Source: CAD feature listing. Evaluate the final solid. Frame: model axes, mm. A direction names the side the tool comes from. Give positions to 0.01 mm unless a question says otherwise; leave off trailing zeros. Order: outer loops, then holes, each group sorted by start corner. A loop starts at its lowest first (then second) coordinate and runs counter-clockwise, first axis right, second up. Notation, with made-up numbers: M 80.25,62 L 119.25,62 A23 ccw 119.25,72 Z; hole C 70.25,73.5 d4. An arc over 180 degrees is marked long. Answer as a JSON object with one key per item and string values. Group by question number.
1. Set-up query: faces 5 (the flat face through (37.5, 40, -10)), 6 (the flat face through (41, 122, -3)), 7 (the flat face through (45, 117, 1)). Return all of +Z, -Z, +X, -X, +Y, -Y with unobstructed straight access to the full face (end or side cutting, diameter ignored); none if empty.
2. Section query C-C (z = -20.5). Output: boundary loops of the cut face in (x, y).
3. Section query B-B (x = 54). Output: boundary loops of the cut face in (y, z), plus the area to 3 significant figures.
4. Material intervals for L1, parallel to Y at x = 50.5, z = 1.75; L2, parallel to Z at x = 24, y = 7; L3, parallel to X at y = 113, z = 4, sorted ascending. Write a range as [from, to].
5. Section query D-D (y = 24). Output: boundary loops of the cut face in (x, z), plus the area to 3 significant figures.
6. Pull-direction query (Y, two-part tool) for faces 1 (the flat face through (40, 0, 2)), 2 (the flat face through (41, 92, -2)), 3 (the flat face through (63, 82, 2)), 4 (the flat face through (0, 40, 2)); classes: +Y half, -Y half, draft (parallel to the pull), parting line (faces both ways), or undercut.
7. Pin query (flat end, axial travel): P1, Ø4, axis at y = 94.5, z = -2, coming from the -X side; P2, Ø2.5, axis at x = 63, z = 3.5, coming from the +Y side; P3, Ø0.9, axis at x = 43, z = -2, coming from the -Y side; P4, Ø12, axis at x = 45.5, z = -7, coming from the +Y side. Return the tip coordinate at first contact, or that it passes through.
8. Section query A-A (y = 40). Output: boundary loops of the cut face in (x, z), plus the area to 3 significant figures.
from build123d import *

# Parameters (mm, degrees)
SKETCH1_W           = 82
SKETCH1_H           = 82
BOSS_EXTRUDE1_DEPTH = 5
SKETCH2_W           = 8
SKETCH2_H           = 5
BOSS_EXTRUDE2_DEPTH = 10
SKETCH4_W           = 8
SKETCH4_H           = 8
BOSS_EXTRUDE4_DEPTH = 60
CUT_REVOLVE1_ANGLE  = 180
SKETCH6_W           = 7
SKETCH6_H           = 25
REVOLVE1_ANGLE      = 180


with BuildPart() as part:
    # Sketch1 → Boss-Extrude1 (new body)
    with BuildSketch(Plane.XY):
        with Locations((41, 41)):
            Rectangle(SKETCH1_W, SKETCH1_H)
    extrude(amount=BOSS_EXTRUDE1_DEPTH)

    # Sketch2 → Boss-Extrude2 (add)
    with BuildSketch(Plane(origin=(0, 82, 0), x_dir=(1, 0, 0), z_dir=(0, 1, 0))):
        with Locations((41, -2.5)):
            Rectangle(SKETCH2_W, SKETCH2_H)
    extrude(amount=BOSS_EXTRUDE2_DEPTH)

    # Sketch4 → Boss-Extrude4 (add)
    with BuildSketch(Plane(origin=(0, 92, 0), x_dir=(1, 0, 0), z_dir=(0, 1, 0))):
        with Locations((41, -1)):
            Rectangle(SKETCH4_W, SKETCH4_H)
    extrude(amount=BOSS_EXTRUDE4_DEPTH)

    # Sketch5 → Cut-Revolve1 (revolve, cut)
    with BuildSketch(Plane(origin=(0, 152, 0), x_dir=(1, 0, 0), z_dir=(0, 1, 0))):
        with BuildLine():
            Line((38.25, -1), (43.75, -1))
            ThreePointArc((43.75, -1), (41, -3.75), (38.25, -1))
        make_face()
    revolve(axis=Axis((38.25, 152, 1), (1, 0, 0)), revolution_arc=CUT_REVOLVE1_ANGLE, mode=Mode.SUBTRACT)

    # Sketch6 → Revolve1 (revolve)
    with BuildSketch(Plane(origin=(0, 0, 0), x_dir=(-1, 0, 0), z_dir=(0, 0, -1))):
        with Locations((-41, 27.5)):
            Rectangle(SKETCH6_W, SKETCH6_H)
    revolve(axis=Axis((37.5, 40, 0), (1, 0, 0)), revolution_arc=REVOLVE1_ANGLE)


solid = part.part
Answer sheet:
{
 "1": {"face 5": "-Z, -X, -Y", "face 6": "-Z, +X, -X, +Y", "face 7": "+Z, -Z, +X, +Y"},
 "2": {"outline": "M 37.5,25.69 L 44.5,25.69 L 44.5,54.31 L 37.5,54.31 Z"},
 "3": {"outline": "M 0,0 L 82,0 L 82,5 L 0,5 Z", "area": "410 mm^2"},
 "4": {"L1": "[0, 82]", "L2": "[0, 5]", "L3": "[37, 45]"},
 "5": {"outline": "M 0,0 L 37.5,0 L 37.5,-19.21 L 44.5,-19.21 L 44.5,0 L 82,0 L 82,5 L 0,5 Z", "area": "544 mm^2"},
 "6": {"face 1": "-Y half", "face 2": "undercut", "face 3": "+Y half", "face 4": "draft"},
 "7": {"P1": "x = 37", "P2": "y = 82", "P3": "y = 15.05", "P4": "y = 152"},
 "8": {"outline": "M 0,0 L 37.5,0 L 37.5,-25 L 44.5,-25 L 44.5,0 L 82,0 L 82,5 L 0,5 Z", "area": "585 mm^2"}
}
